Verification items for this drawing (mm, ordinates from the low corner). Round coordinates to 2 decimals unless told otherwise and drop trailing zeros. Loops run counter-clockwise (first coordinate to the right, second up) from the corner with the lowest first, then second, coordinate; pieces in that order, holes last. Notation, with made-up numbers: (27.5, 8.5) -> (71.5, 8.5) arc R26 ccw to (71.5, 40.5) -> close; hole circle Ø11 at (86, 55). An arc over 180 degrees is marked (long way). Use a Markdown table: item, result. Add a question column.
Q1. Material ranges on L1, parallel to X at y = 152.4, z = 1.2 (1 decimal); L2, parallel to Y at x = 21, z = 0.75; L3, parallel to X at y = 203.2, z = 1.2, recorded low to high.
Q2. Sectioned sample at C-C, the plane y = 59.5. Enter the section's corners in (x, z) (3 decimals).
Q3. Sectioned sample at A-A, the plane x = 200. Enter the section's corners in (y, z) (3 decimals).
Q4. Sectioned sample at B-B, the plane z = 0.5. Give the number of separate pieces and of enclosed holes in the cut face, then the cut area to 3 significant figures.
Q5. Gauge pin test, flat ends, axial feed: P1, Ø4, axis at x = 41.275, y = 127, coming from the +Z side; P2, Ø1.6, axis at y = 133, z = 1, coming from the -X side (3 decimals). Record the tip position at first contact, or that the pin passes through.
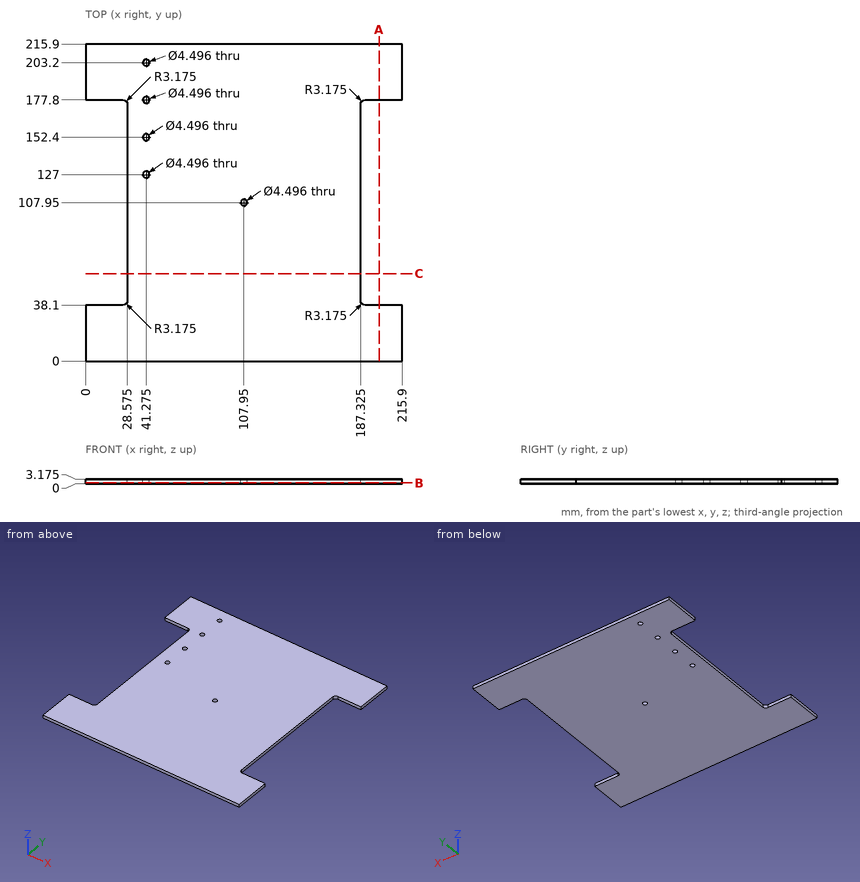
Values:
| question | item | result |
|---|---|---|
| 1 | L1 | 28.6 to 39, 43.5 to 187.3 |
| 1 | L2 | 0 to 38.1, 177.8 to 215.9 |
| 1 | L3 | 0 to 39.03, 43.52 to 215.9 |
| 2 | outline | (28.575, 0) -> (187.325, 0) -> (187.325, 3.175) -> (28.575, 3.175) -> close |
| 3 | outline | (0, 0) -> (38.1, 0) -> (38.1, 3.175) -> (0, 3.175) -> close; (177.8, 0) -> (215.9, 0) -> (215.9, 3.175) -> (177.8, 3.175) -> close |
| 4 | separate pieces | 1 |
| 4 | enclosed holes | 5 |
| 4 | area | 38,600 mm^2 |
| 5 | P1 | through |
| 5 | P2 | x = 28.575 |
